Input: part model. Units: mm. Frame: model coordinates. A direction names the side the tool comes from. Give positions to 0.01 mm unless a question says otherwise; leave off trailing zeros. Write each loop counter-clockwise with the first axis right and the second up, starting at its lowest first coordinate (ties: lowest second). Pieces come first, ordered by that corner, then holes.
```python
from build123d import *

# Parameters (mm, degrees)
SKETCH_1_W          = 26.5
SKETCH_1_H          = 26.5
SKETCH_1_W_2        = 20.5
SKETCH_1_H_2        = 20.5
EXTRUDE_3_DEPTH     = 50
SKETCH_2_R          = 2.65
SKETCH_2_W          = 21.75
SKETCH_2_H          = 50
EXTRUDE_4_DEPTH     = 5
CUT_EXTRUDE_1_DEPTH = 67.537583365
SKETCH_4_R          = 2.65
CUT_EXTRUDE_2_DEPTH = 71.736306095
FILLET_1_R          = 5


with BuildPart() as part:
    # 草图1 → 凸台-拉伸3 (new body)
    with BuildSketch(Plane.XY):
        Rectangle(SKETCH_1_W, SKETCH_1_H)
        Rectangle(SKETCH_1_W_2, SKETCH_1_H_2, mode=Mode.SUBTRACT)
    extrude(amount=EXTRUDE_3_DEPTH)

    # 草图2 → 凸台-拉伸4 (add)
    # profile 1 of 2: a face of its own
    with BuildSketch(Plane(origin=(0, 13.25, 0), x_dir=(1, 0, 0), z_dir=(0, 1, 0))):
        Polygon((-13.25, -50), (-13.25, -25), (-13.25, 0), (-35, 0), (-35, -50), align=None)
        with Locations(Location((-28, -41.5, 0), (0, 0, 270))):
            Circle(SKETCH_2_R, mode=Mode.SUBTRACT)
        with Locations(Location((-28, -8.5, 0), (0, 0, 270))):
            Circle(SKETCH_2_R, mode=Mode.SUBTRACT)
    # profile 2 of 2: a face of its own
    with BuildSketch(Plane(origin=(0, 13.25, 0), x_dir=(1, 0, 0), z_dir=(0, 1, 0))):
        with Locations((24.125, -25)):
            Rectangle(SKETCH_2_W, SKETCH_2_H)
        with Locations(Location((28, -41.5, 0), (0, 0, 270))):
            Circle(SKETCH_2_R, mode=Mode.SUBTRACT)
        with Locations(Location((28, -8.5, 0), (0, 0, 270))):
            Circle(SKETCH_2_R, mode=Mode.SUBTRACT)
    extrude(amount=-EXTRUDE_4_DEPTH)

    # 草图3 → 切除-拉伸1 (cut, through all)
    with BuildSketch(Plane(origin=(0, 13.25, 0), x_dir=(1, 0, 0), z_dir=(0, 1, 0))):
        with BuildLine():
            ThreePointArc((2.65, -15), (1.87383297, -13.12616703), (0, -12.35))
            Line((0, -12.35), (0, -17.65))
            ThreePointArc((0, -17.65), (1.87383297, -16.87383297), (2.65, -15))
        make_face()
        with BuildLine():
            Line((0, -17.65), (0, -12.35))
            ThreePointArc((0, -12.35), (-2.65, -15), (0, -17.65))
        make_face()
        with BuildLine():
            ThreePointArc((2.65, -35), (1.87383297, -33.12616703), (0, -32.35))
            Line((0, -32.35), (0, -37.65))
            ThreePointArc((0, -37.65), (1.87383297, -36.87383297), (2.65, -35))
        make_face()
        with BuildLine():
            Line((0, -37.65), (0, -32.35))
            ThreePointArc((0, -32.35), (-2.65, -35), (0, -37.65))
        make_face()
    extrude(amount=-CUT_EXTRUDE_1_DEPTH, mode=Mode.SUBTRACT)

    # 草图4 → 切除-拉伸2 (cut, through all)
    with BuildSketch(Plane.ZY.offset(13.25)):
        with Locations((15, 0)):
            Circle(SKETCH_4_R)
        with Locations((35, 0)):
            Circle(SKETCH_4_R)
    extrude(amount=-CUT_EXTRUDE_2_DEPTH, mode=Mode.SUBTRACT)

    # 圆角1
    fillet_1_edges = [part.edges().sort_by_distance(p)[0] for p in [
        (-13.25, 8.25, 25),
        (13.25, 8.25, 25),
    ]]
    fillet(fillet_1_edges, radius=FILLET_1_R)


solid = part.part
```
Item 1: Set-up query: faces 5 (the flat face through (10.25, 0, 25)), 6 (the flat face through (27, 8.25, 25)), 7 (the flat face through (-13.25, -5, 25)), 8 (the cylindrical face through (-27.883, 10.785, 5.853)). Return all of +Z, -Z, +X, -X, +Y, -Y with unobstructed straight access to the full face (end or side cutting, diameter ignored); none if empty.
Item 2: Section B-B (z = 8.5). Return loops of the section in (x, y).
Item 3: Pin query (flat end, axial travel): pin 1 (13 mm diameter, centred on y = -1, z = 37.5, fed in from +X); pin 2 (1.5 mm diameter, centred on y = 6.5, z = 8.5, fed in from -X); pin 3 (5 mm diameter, centred on x = -28, z = 8.5, fed in from +Y); pin 4 (6 mm diameter, centred on y = 0, z = 35, fed in from -X). Return the tip coordinate at first contact, or that it passes through.
Item 4: Section D-D (z = 20). Return loops of the section in (x, y), and give its area (3 significant figures).
Item 5: Section C-C (x = -28). Return loops of the section in (y, z), and give its area (3 significant figures).
Item 6: Ray query, line 1 (X direction, y = 9.9, z = 41.5); line 2 (X direction, y = 10.3, z = 41.5); line 3 (X direction, y = 9.75, z = 2). Return the intervals inside material, ascending.
Item 7: Section A-A (y = 9.5). Return loops of the section in (x, z), and give its area (3 significant figures).
Item 8: Mould query, pull axis Y, two halves, no side actions, for faces 1 (the cylindrical face through (11.729, 0.117, 32.353)), 2 (the flat face through (-10.25, 0, 25)), 3 (the cylindrical face through (-14.75, 6.82, 24.65)), 4 (the cylindrical face through (28.117, 10.785, 38.853)). Classes: +Y half, -Y half, draft (parallel to the pull), parting line (faces both ways), or undercut.
Solved:
1. face 5: +Z, -Z
1. face 6: +Z, -Z, +X, -Y
1. face 7: +Z, -Z, -X, -Y
1. face 8: +Y, -Y
2. outline: (-35, 8.25) - (-30.65, 8.25) - (-30.65, 13.25) - (-35, 13.25) - close; (-25.35, 8.25) - (-18.25, 8.25) arc R5 cw to (-13.25, 3.25) - (-13.25, -13.25) - (13.25, -13.25) - (13.25, 3.25) arc R5 cw to (18.25, 8.25) - (25.35, 8.25) - (25.35, 13.25) - (-25.35, 13.25) - close; (30.65, 8.25) - (35, 8.25) - (35, 13.25) - (30.65, 13.25) - close; hole (-10.25, -10.25) - (10.25, -10.25) - (10.25, 10.25) - (-10.25, 10.25) - close
3. pin 1: stops at x = 13.78
3. pin 2: stops at x = -15.25
3. pin 3: passes through
3. pin 4: stops at x = -13.25
4. outline: (-35, 8.25) - (-18.25, 8.25) arc R5 cw to (-13.25, 3.25) - (-13.25, -13.25) - (13.25, -13.25) - (13.25, 3.25) arc R5 cw to (18.25, 8.25) - (35, 8.25) - (35, 13.25) - (-35, 13.25) - close; hole (-10.25, -10.25) - (10.25, -10.25) - (10.25, 10.25) - (-10.25, 10.25) - close
4. area: 510 mm2
5. outline: (8.25, 0) - (13.25, 0) - (13.25, 5.85) - (8.25, 5.85) - close; (8.25, 11.15) - (13.25, 11.15) - (13.25, 38.85) - (8.25, 38.85) - close; (8.25, 44.15) - (13.25, 44.15) - (13.25, 50) - (8.25, 50) - close
5. area: 197 mm2
6. line 1: x = -35 to -30.65, -25.35 to -10.25, 10.25 to 25.35, 30.65 to 35
6. line 2: x = -35 to -30.65, -25.35 to 25.35, 30.65 to 35
6. line 3: x = -35 to -10.25, 10.25 to 35
7. outline: (-35, 0) - (-10.25, 0) - (-10.25, 50) - (-35, 50) - close; (10.25, 0) - (35, 0) - (35, 50) - (10.25, 50) - close; hole circle Ø5.3 at (-28, 8.5); hole circle Ø5.3 at (-28, 41.5); hole circle Ø5.3 at (28, 8.5); hole circle Ø5.3 at (28, 41.5)
7. area: 2,390 mm2
8. face 1: undercut
8. face 2: undercut
8. face 3: -Y half
8. face 4: draft
